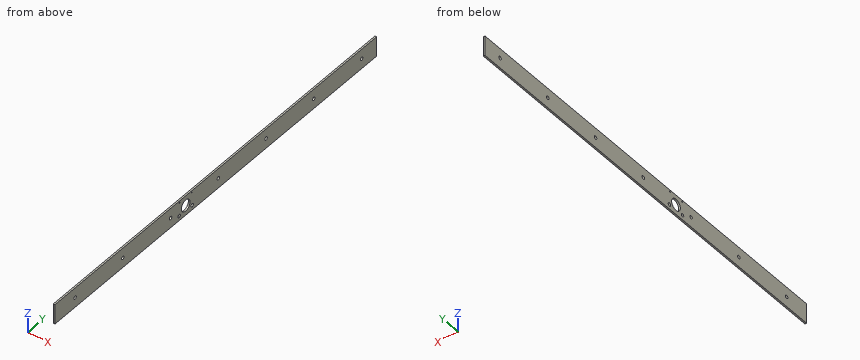
```python
from build123d import *

# Parameters (mm, degrees)
F1_DEPTH = 812.8
F2_R     = 10.9982
F2_R_2   = 1.0922
F3_DEPTH = 25.4
F4_R     = 3.175
F5_DEPTH = 25.4


with BuildPart() as f1:
    # F0 (on Front) → F1 (new body)
    with BuildSketch(Plane.XZ):
        Polygon((0, -3.175), (0, 0), (0, 34.925), (-3.175, 34.925), (-3.175, -3.175), align=None)
    extrude(amount=F1_DEPTH)

    # F2 (on face) → F3 (cut)
    with BuildSketch(Plane.YZ):
        with Locations((-482.6, 15.875)):
            Circle(F2_R)
        with BuildLine():
            ThreePointArc((-497.0280745814, 3.3178743146), (-496.2211647499, 4.3977088788), (-495.935, 5.715))
            ThreePointArc((-495.935, 5.715), (-501.5319671306, 7.7679735064), (-498.5899292713, 2.5828838723))
            ThreePointArc((-498.5899292713, 2.5828838723), (-498.664634248, 4.4872772922), (-497.0018, 3.556))
            ThreePointArc((-497.0018, 3.556), (-497.0083885174, 3.4362145714), (-497.0280745814, 3.3178743146))
        make_face()
        with BuildLine():
            ThreePointArc((-497.0018, 3.556), (-498.664634248, 4.4872772922), (-498.5899292713, 2.5828838723))
            ThreePointArc((-498.5899292713, 2.5828838723), (-497.7580944097, 2.8422006205), (-497.0280745814, 3.3178743146))
            ThreePointArc((-497.0280745814, 3.3178743146), (-497.0083885174, 3.4362145714), (-497.0018, 3.556))
        make_face()
        with BuildLine():
            ThreePointArc((-497.0280745814, 3.3178743146), (-497.7580944097, 2.8422006205), (-498.5899292713, 2.5828838723))
            ThreePointArc((-498.5899292713, 2.5828838723), (-497.6289444769, 2.5677570135), (-497.0280745814, 3.3178743146))
        make_face()
        with BuildLine():
            ThreePointArc((-466.6100707287, 2.5828838723), (-464.0370264936, 3.2930328694), (-462.915, 5.715))
            ThreePointArc((-462.915, 5.715), (-467.4072911212, 8.6038352501), (-468.1719254186, 3.3178743146))
            ThreePointArc((-468.1719254186, 3.3178743146), (-467.2257854286, 4.6416114826), (-466.0138, 3.556))
            ThreePointArc((-466.0138, 3.556), (-466.1747227078, 2.985365752), (-466.6100707287, 2.5828838723))
        make_face()
        with BuildLine():
            ThreePointArc((-466.0138, 3.556), (-467.2257854286, 4.6416114826), (-468.1719254186, 3.3178743146))
            ThreePointArc((-468.1719254186, 3.3178743146), (-467.4419055903, 2.8422006205), (-466.6100707287, 2.5828838723))
            ThreePointArc((-466.6100707287, 2.5828838723), (-466.1747227078, 2.985365752), (-466.0138, 3.556))
        make_face()
        with BuildLine():
            ThreePointArc((-466.6100707287, 2.5828838723), (-467.4419055903, 2.8422006205), (-468.1719254186, 3.3178743146))
            ThreePointArc((-468.1719254186, 3.3178743146), (-467.5710555231, 2.5677570135), (-466.6100707287, 2.5828838723))
        make_face()
        with Locations((-498.094, 31.369)):
            Circle(F2_R_2)
        with Locations((-467.106, 31.369)):
            Circle(F2_R_2)
    extrude(amount=-F3_DEPTH, mode=Mode.SUBTRACT)

    # F4 (on face) → F5 (cut)
    with BuildSketch(Plane(origin=(-3.175, 0, 0), x_dir=(0, -1, 0), z_dir=(-1, 0, 0))):
        with Locations((762, 15.875)):
            Circle(F4_R)
        with Locations((641.3500135583, 15.9321981283)):
            Circle(F4_R)
        with Locations((520.7000271167, 15.9893962565)):
            Circle(F4_R)
        with Locations((400.050040675, 16.0465943848)):
            Circle(F4_R)
        with Locations((279.4000542333, 16.103792513)):
            Circle(F4_R)
        with Locations((158.7500677917, 16.1609906413)):
            Circle(F4_R)
        with Locations((38.10008135, 16.2181887695)):
            Circle(F4_R)
    extrude(amount=-F5_DEPTH, mode=Mode.SUBTRACT)


solid = f1.part
```
The listing builds one solid part. Answer for the finished solid, in the listing's coordinates (mm). Coordinates: 2 decimals unless noted, no trailing zeros. Write each loop counter-clockwise with the first axis right and the second up, starting at its lowest first coordinate (ties: lowest second). Pieces come first, ordered by that corner, then holes.
Q1. Section B-B, the plane x = -2.3 is taken. Give the number of separate pieces and of enclosed holes in the cut face, then the cut area to 3 significant figures.
Returned:
separate pieces: 1
enclosed holes: 12
area: 30,300 mm2
Q2. Section A-A, the plane y = -482.6 is taken. Write down the section's boundary in (x, z) (3 decimals).
Returned:
outline: (-3.175, -3.175) - (0, -3.175) - (0, 4.877) - (-3.175, 4.877) - close; (-3.175, 26.873) - (0, 26.873) - (0, 34.925) - (-3.175, 34.925) - close
Q3. Given P1, Ø5.5, axis at y = -520.7, z = 15.99, coming from the -X side (1 decimal), flat-ended and moving along its own axis, determine where the tip first touches the part or whether it passes through.
Returned:
P1: passes through
Q4. Find the intervals of material crossed by line 1 along Y through (x, z) = (-1.9, 3.5); line 2 along Z through (x, y) = (-2.15, -762) (3 decimals); line 3 along Y through (x, z) = (-0.4, 7), in increasing order.
Returned:
line 1: y = -812.8 to -501.38, -496.84 to -468.36, -463.82 to 0
line 2: z = -3.175 to 12.7, 19.05 to 34.925
line 3: y = -812.8 to -502.01, -496.21 to -489.1, -476.1 to -468.99, -463.19 to 0
